```python
from build123d import *

# Parameters (mm, degrees)
F0_W           = 5
F0_H           = 15
F0_H_2         = 5
F0_R           = 1.663624267
F0_W_2         = 15
F1_DEPTH       = 3
F2_R           = 2
F4_D           = 3
F6_D           = 2
F6_CBORE_D     = 3
F6_CBORE_DEPTH = 1.5


with BuildPart() as f1:
    # F0 (on Front) → F1 (new body)
    with BuildSketch(Plane.XZ):
        with Locations((0, -10)):
            Rectangle(F0_W, F0_H)
        Rectangle(F0_W, F0_H_2)
        Circle(F0_R, mode=Mode.SUBTRACT)
        with Locations((10, 0)):
            Rectangle(F0_W_2, F0_H_2)
        with Locations((-10, 0)):
            Rectangle(F0_W_2, F0_H_2)
        with Locations((0, 10)):
            Rectangle(F0_W, F0_H)
    extrude(amount=F1_DEPTH)

    # F2
    f2_edges = [f1.edges().sort_by_distance(p)[0] for p in [
        (17.5, -1.5, 2.5),
        (17.5, -1.5, -2.5),
        (2.5, -1.5, -17.5),
        (-17.5, -1.5, 2.5),
        (2.5, -1.5, 17.5),
        (-2.5, -1.5, 17.5),
        (-2.5, -1.5, -17.5),
        (-17.5, -1.5, -2.5),
        (-2.5, -1.5, 2.5),
        (2.5, -1.5, -2.5),
        (2.5, -1.5, 2.5),
        (-2.5, -1.5, -2.5),
    ]]
    fillet(f2_edges, radius=F2_R)

    # F4 (through all)
    with Locations(Plane.XZ.offset(3)):
        with Locations((-15, 0), (0, 15), (15, 0), (0, -15)):
            Hole(F4_D / 2)

    # F6 (through all)
    with Locations(Plane.XZ.offset(3)):
        with Locations((0, 9), (9, 0), (0, -9), (-9, 0)):
            CounterBoreHole(F6_D / 2, F6_CBORE_D / 2, F6_CBORE_DEPTH)


solid = f1.part
```
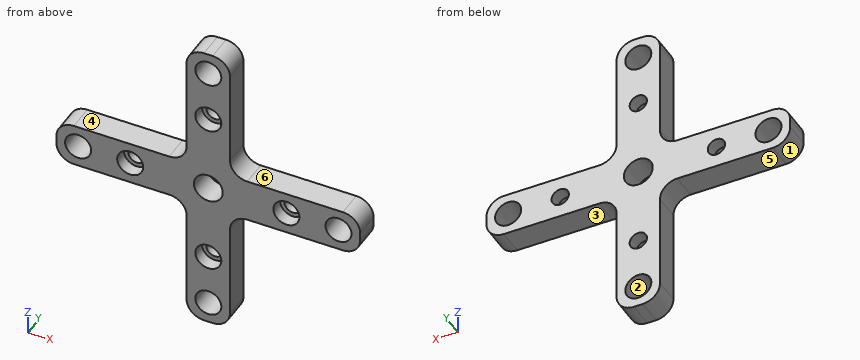
Work out the finished part from the listing and answer in its coordinate system (mm). Face numbers are marked on the shaded views. A direction names the side the tool comes from. Round coordinates to 2 decimals unless told otherwise and drop trailing zeros. Write each loop counter-clockwise with the first axis right and the second up, starting at its lowest first coordinate (ties: lowest second). Pieces come first, ordered by that corner, then holes.
1) Consider probe 1 along Z at (x, y) = (0, -0.25); probe 2 along Z at (x, y) = (-9, -2.5); probe 3 along Z at (x, y) = (0, -1.9). Determine where each line is inside the solid, lowest interval first.
2) A cutting plane is placed at B-B on x = 0. Give the number of separate pieces and of enclosed holes in the cut face, and give its area (3 significant figures).
3) Flat-ended cylindrical pins translate along their axes: P1, Ø0.9, axis at x = 8.5, y = -2, coming from the +Z side; P2, Ø1.5, axis at y = -0.5, z = 11.5, coming from the +X side; P3, Ø2.5, axis at x = 0, z = -9, coming from the -Y side. Find the tip coordinate at first contact, or state that the pin passes through.
4) Which of the six approach directions +Z, -Z, +X, -X, +Y, -Y give full straight-line access (tool end or side, diameter ignored) to the marked faces 4, 5 and 6?
5) A cutting plane is placed at A-A on z = -9. Determine the outline of the cut face in (x, y).
6) A cutting plane is placed at D-D on x = -15. Determine the outline of the cut face in (y, z).
7) Determine the mould class of the marked faces 1, 2 and 3 for opening direction X: pulls with the +X half, pulls with the -X half, needs draft (parallel to the pull), parting line crosses it, or undercut.
Entries:
1. probe 1: z = -17.5 to -16.5, -13.5 to -10, -8 to -1.66, 1.66 to 8, 10 to 13.5, 16.5 to 17.5
1. probe 2: z = -2.5 to -1.5, 1.5 to 2.5
1. probe 3: z = -17.5 to -16.5, -13.5 to -10.5, -7.5 to -1.66, 1.66 to 7.5, 10.5 to 13.5, 16.5 to 17.5
2. separate pieces: 6
2. enclosed holes: 0
2. area: 62.0 mm2
3. P1: stops at z = 2.5
3. P2: stops at x = 2.5
3. P3: stops at y = -1.5
4. face 4: +Z, -X, +Y, -Y
4. face 5: -Z, -X, +Y, -Y
4. face 6: +Z, +X, +Y, -Y
5. outline: (-2.5, -3) - (-1.5, -3) - (-1.5, -1.5) - (-1, -1.5) - (-1, 0) - (-2.5, 0) - close; (1, -1.5) - (1.5, -1.5) - (1.5, -3) - (2.5, -3) - (2.5, 0) - (1, 0) - close
6. outline: (-3, -2.5) - (0, -2.5) - (0, -1.5) - (-3, -1.5) - close; (-3, 1.5) - (0, 1.5) - (0, 2.5) - (-3, 2.5) - close
7. face 1: pulls with the -X half
7. face 2: undercut
7. face 3: needs draft
